from build123d import *

# Parameters (mm, degrees)
SKETCH_1_W          = 200
SKETCH_1_H          = 115
F_35MM_DEPTH        = 35
SHELL_3_T           = 1.5
SKETCH_2_W          = 165
SKETCH_2_H          = 100
CUT_EXTRUDE_7_DEPTH = 1.5
SKETCH_3_W          = 16
SKETCH_3_H          = 10
CUT_EXTRUDE_8_DEPTH = 1.5
SKETCH_4_W          = 23
SKETCH_4_H          = 12
CUT_EXTRUDE_9_DEPTH = 1.5
EXTRUDE_1_DEPTH     = 13
EXTRUDE_2_DEPTH     = 2
FILLET_2_R          = 1


with BuildPart() as part:
    # 草图1 → 凸台-拉伸35mm (new body)
    with BuildSketch(Plane(origin=(0, 0, 0), x_dir=(1, 0, 0), z_dir=(0, 1, 0))):
        Rectangle(SKETCH_1_W, SKETCH_1_H)
    extrude(amount=F_35MM_DEPTH)

    # 抽壳3
    shell_3_openings = [part.faces().sort_by_distance(p)[0] for p in [
        (0, 0, 0),
    ]]
    offset(amount=SHELL_3_T, openings=shell_3_openings, kind=Kind.INTERSECTION)

    # 草图2 → 切除-拉伸7 (cut)
    with BuildSketch(Plane(origin=(0, 35, 0), x_dir=(1, 0, 0), z_dir=(0, 1, 0))):
        Rectangle(SKETCH_2_W, SKETCH_2_H)
    extrude(amount=CUT_EXTRUDE_7_DEPTH, mode=Mode.SUBTRACT)

    # 草图3 → 切除-拉伸8 (cut)
    with BuildSketch(Plane(origin=(-100, 0, 0), x_dir=(0, 0, -1), z_dir=(1, 0, 0))):
        with Locations((12, 22.5)):
            Rectangle(SKETCH_3_W, SKETCH_3_H)
    extrude(amount=-CUT_EXTRUDE_8_DEPTH, mode=Mode.SUBTRACT)

    # 草图4 → 切除-拉伸9 (cut)
    with BuildSketch(Plane.ZY.offset(-100)):
        with Locations((0, 17.5)):
            Rectangle(SKETCH_4_W, SKETCH_4_H)
    extrude(amount=-CUT_EXTRUDE_9_DEPTH, mode=Mode.SUBTRACT)

    # 草图6 → 凸台-拉伸1 (add)
    with BuildSketch(Plane(origin=(0, 35, 0), x_dir=(-1, 0, 0), z_dir=(0, -1, 0))):
        Polygon((-95.25, 52.7), (-85.25, 52.7), (-85.25, 54.2), (-96.75, 54.2), (-96.75, 42.7), (-95.25, 42.7), align=None)
        Polygon((-96.75, -42.7), (-95.25, -42.7), (-95.25, -52.7), (-85.25, -52.7), (-85.25, -54.2), (-96.75, -54.2), align=None)
        Polygon((85.25, -52.7), (85.25, -54.2), (96.75, -54.2), (96.75, -42.7), (95.25, -42.7), (95.25, -52.7), align=None)
        Polygon((85.25, 52.7), (85.25, 54.2), (96.75, 54.2), (96.75, 42.7), (95.25, 42.7), (95.25, 52.7), align=None)
    extrude(amount=EXTRUDE_1_DEPTH)

    # 草图7 → 凸台-拉伸2 (add)
    with BuildSketch(Plane.ZY.offset(-100)):
        Polygon((13, 15.5), (11.5, 15.5), (11.5, 11.5), (7.5, 11.5), (7.5, 10), (13, 10), align=None)
        Polygon((-7.5, 23.5), (-7.5, 25), (-13, 25), (-13, 19.5), (-11.5, 19.5), (-11.5, 23.5), align=None)
        Polygon((7.5, 23.5), (7.5, 25), (13, 25), (13, 19.5), (11.5, 19.5), (11.5, 23.5), align=None)
        Polygon((-7.5, 11.5), (-7.5, 10), (-13, 10), (-13, 15.5), (-11.5, 15.5), (-11.5, 11.5), align=None)
    extrude(amount=EXTRUDE_2_DEPTH)

    # 圆角2
    fillet_2_edges = [part.edges().sort_by_distance(p)[0] for p in [
        (101.5, 36.5, 0),
        (0, 36.5, -59),
        (100, 17.5, 57.5),
        (-101.5, 36.5, 0),
        (-101.5, 18.25, -59),
        (101.5, 18.25, -59),
        (-101.5, 18.25, 59),
        (0, 36.5, 59),
    ]]
    fillet(fillet_2_edges, radius=FILLET_2_R)


solid = part.part
Here's how the part is built. I have some questions about the finished solid (model axes, mm). A direction names the side the tool comes from. Give positions to 0.01 mm unless a question says otherwise; leave off trailing zeros. Loops run counter-clockwise (first coordinate to the right, second up) from the corner with the lowest first, then second, coordinate; pieces in that order, holes last. Notation, with made-up numbers: (39.25, -35.75) -> (44.25, -35.75) arc R19 ccw to (44.25, -4.75) -> close; hole circle Ø3 at (24.5, -14.75). An arc over 180 degrees is marked (long way). One line per item, written item: value.
Q1. If I drill on line 1 along Z through (x, y) = (85.5, 29); line 2 along X through (y, z) = (2, -52.5); line 3 along Z through (x, y) = (35.5, 21.5), over which ranges is the centre line in solid material (lowest first)?
Answers follow:
line 1: -59 to -57.5, -54.2 to -52.7, 52.7 to 54.2, 57.5 to 59
line 2: -101.5 to -100, 100 to 101.5
line 3: -59 to -57.5, 57.5 to 59
Q2. Suppose I cut it at A-A on x = -5. Please give me the cut outline in (y, z), then the cut area to 3 significant figures.
Answers follow:
outline: (0, -59) -> (35.5, -59) arc R1 ccw to (36.5, -58) -> (36.5, -50) -> (35, -50) -> (35, -57.5) -> (0, -57.5) -> close; (0, 57.5) -> (35, 57.5) -> (35, 50) -> (36.5, 50) -> (36.5, 58) arc R1 ccw to (35.5, 59) -> (0, 59) -> close
area: 132 mm^2
Q3. On a 3-axis mill with a long thin cutter (end or side, diameter ignored), from which of +Z, -Z, +X, -X, +Y, -Y can I reach the whole of each face in a straight line? I mean faces 1 (the face through (98, 12, 12)), 2 (the face through (-1, 18, 59)). Say none if no direction works.
Answers follow:
face 1: -Y
face 2: +Z, +X, -X, +Y, -Y
Q4. I'm going to push flat-ended pins straight in: pin 1 Ø9 at (x, z) = (94, 50) entering from -Y; pin 2 Ø1 at (x, z) = (98.5, -9.5) entering from -Y; pin 3 Ø0.8 at (y, z) = (36, 15.5) entering from -X (3 decimals); pin 4 Ø10 at (x, z) = (39, -40.5) entering from +Y. Where does each tip first touch, or does it pass through?
Answers follow:
pin 1: y = 22
pin 2: y = 10
pin 3: x = -101.495
pin 4: through
Q5. Suppose I cut it at B-B on z = -27. Please give me the cut outline in (x, y), then the cut area to 3 significant figures.
Answers follow:
outline: (-101.5, 0) -> (-100, 0) -> (-100, 35) -> (-82.5, 35) -> (-82.5, 36.5) -> (-100.5, 36.5) arc R1 ccw to (-101.5, 35.5) -> close; (82.5, 35) -> (100, 35) -> (100, 0) -> (101.5, 0) -> (101.5, 35.5) arc R1 ccw to (100.5, 36.5) -> (82.5, 36.5) -> close
area: 162 mm^2
Q6. Suppose I cut it at D-D on z = 1. Please give me the cut outline in (x, y).
Answers follow:
outline: (-101.5, 0) -> (-100, 0) -> (-100, 35) -> (-82.5, 35) -> (-82.5, 36.5) -> (-100.5, 36.5) arc R1 ccw to (-101.5, 35.5) -> close; (82.5, 35) -> (100, 35) -> (100, 23.5) -> (101.5, 23.5) -> (101.5, 35.5) arc R1 ccw to (100.5, 36.5) -> (82.5, 36.5) -> close; (100, 0) -> (101.5, 0) -> (101.5, 11.5) -> (100, 11.5) -> close
Q7. Suppose I cut it at C-C on y = 8. Please give me the cut outline in (x, z), then the cut area to 3 significant figures.
Answers follow:
outline: (-101.5, -58) arc R1 ccw to (-100.5, -59) -> (100.5, -59) arc R1 ccw to (101.5, -58) -> (101.5, 59) -> (-100.5, 59) arc R1 ccw to (-101.5, 58) -> close; hole (-100, -57.5) -> (100, -57.5) -> (100, 56.5) arc R1 ccw to (99, 57.5) -> (-100, 57.5) -> close
area: 954 mm^2
